Verification items for the finished model (mm, model axes). Coordinates: 2 decimals unless noted, no trailing zeros. Order: outer loops, then holes, each group sorted by start corner. A loop starts at its lowest first (then second) coordinate and runs counter-clockwise, first axis right, second up. Notation, with made-up numbers: (-2.75, 62) -> (56.25, 62) arc R16 cw to (56.25, 69) -> close; hole circle Ø4 at (47.25, -40). An arc over 180 degrees is marked (long way). Use CSV: the item, a comma, the result in double quotes. Start each with the question number.
1) Scan lines: line 1 along Y through (x, z) = (59, 2); line 2 along Y through (x, z) = (-2, 1.55). Record each from-to range of solid material in increasing order.
2) Release check for a two-part mould opening along X. For faces 1 (the cylindrical face through (-57.66, 24.39, 1.48)), 2 (the flat face through (-1, 32.5, 1)), 3 (the cylindrical face through (63.5, 31.07, 1.48)), 4 (the cylindrical face through (-63.5, -31.07, 1.48)) record: released by +X, released by -X, zero draft, split by the parting line, or undercut.
3) Sectioned sample at C-C on x = 0. Record the boundary of the cut face in (y, z), then the cut area to 3 significant figures.
4) Sectioned sample at A-A on y = 0. Record the boundary of the cut face in (x, z).
5) Sectioned sample at B-B on z = 0.55. Record the boundary of the cut face in (x, y), then the cut area to 3 significant figures.
Autodesk Fusion 360 part; units mm, degrees
sketch "Sketch1" plane through (0, 0, 0) normal (0, 0, 1) x (1, 0, 0)
  line L0 (-60, 32.5) -> (60, 32.5)
  line L1 (65, 27.5) -> (65, -27.5)
  line L2 (60, -32.5) -> (-60, -32.5)
  line L3 (-65, -27.5) -> (-65, 27.5)
  arc A0 (-60, 32.5) -> (-65, 27.5) centre (-60, 27.5) ccw
  arc A1 (-65, -27.5) -> (-60, -32.5) centre (-60, -27.5) ccw
  arc A2 (65, 27.5) -> (60, 32.5) centre (60, 27.5) ccw
  arc A3 (60, -32.5) -> (65, -27.5) centre (60, -27.5) ccw
  circle A4 centre (-59, 26.5) radius 2.5
  circle A5 centre (-59, -26.5) radius 2.5
  circle A6 centre (59, 26.5) radius 2.5
  circle A7 centre (59, -26.5) radius 2.5
  circle A8 centre (0, 0) radius 3.5
  dimension "d1" = 65
  dimension "d2" = 65
  dimension "d3" = 32.5
  dimension "d4" = 32.5
  dimension "d5" = 5
  dimension "d6" = 5
  dimension "d7" = 5
  dimension "d8" = 5
  dimension "d9" = 5
  dimension "d10" = 6
  dimension "d11" = 6
  dimension "d12" = 5
  dimension "d13" = 6
  dimension "d14" = 6
  dimension "d15" = 5
  dimension "d16" = 6
  dimension "d17" = 6
  dimension "d18" = 5
  dimension "d19" = 6
  dimension "d20" = 6
  dimension "d21" = 7
extrude "Extrude1" add sketch "Sketch1" along normal blind 3
equation "d2 = d1"
equation "d3 = ( 65 / 2 ) * 1 mm"
equation "d4 = d3"
equation "d6 = d5"
equation "d7 = d5"
equation "d8 = d5"
equation "d11 = d10"
equation "d12 = d9"
equation "d13 = d10"
equation "d14 = d10"
equation "d15 = d9"
equation "d16 = d10"
equation "d17 = d10"
equation "d18 = d9"
equation "d19 = d10"
equation "d20 = d10"
Answers follow:
1,line 1,"y = -32.5 to -29, -24 to 24, 29 to 32.5"
1,line 2,"y = -32.5 to -2.87, 2.87 to 32.5"
2,face 1,"undercut"
2,face 2,"zero draft"
2,face 3,"released by +X"
2,face 4,"released by -X"
3,outline,"(-32.5, 0) -> (-3.5, 0) -> (-3.5, 3) -> (-32.5, 3) -> close; (3.5, 0) -> (32.5, 0) -> (32.5, 3) -> (3.5, 3) -> close"
3,area,"174 mm²"
4,outline,"(-65, 0) -> (-3.5, 0) -> (-3.5, 3) -> (-65, 3) -> close; (3.5, 0) -> (65, 0) -> (65, 3) -> (3.5, 3) -> close"
5,outline,"(-65, -27.5) arc R5 ccw to (-60, -32.5) -> (60, -32.5) arc R5 ccw to (65, -27.5) -> (65, 27.5) arc R5 ccw to (60, 32.5) -> (-60, 32.5) arc R5 ccw to (-65, 27.5) -> close; hole circle Ø5 at (-59, -26.5); hole circle Ø5 at (-59, 26.5); hole circle Ø7 at (0, 0); hole circle Ø5 at (59, -26.5); hole circle Ø5 at (59, 26.5)"
5,area,"8,310 mm²"
